Read the model definition and answer for the solid it produces. Units are mm, in the model's axes. Coordinates: 2 decimals unless noted, no trailing zeros. Order: outer loops, then holes, each group sorted by start corner. A loop starts at its lowest first (then second) coordinate and runs counter-clockwise, first axis right, second up. Notation, with made-up numbers: (31.5, -25) - (58.5, -25) arc R14 cw to (58.5, -17) - close; hole circle Ø6 at (69.5, -29). An arc over 180 degrees is marked (long way). Use one line per item in the form item = value.
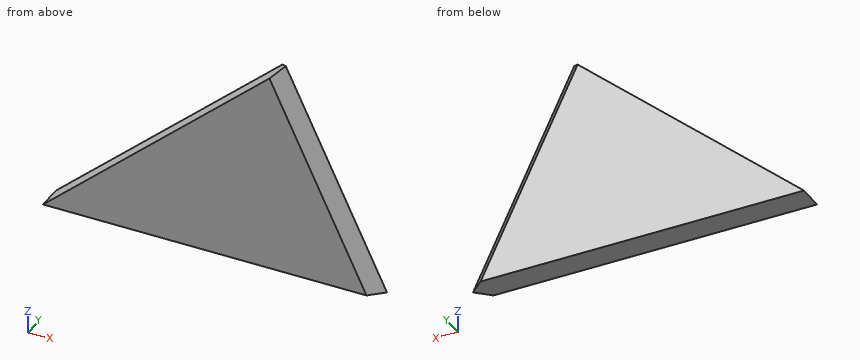
Solid Edge part; units mm, degrees
sketch "Sketch1" plane through (0, 0, 0) normal (0, -1, 0) x (1, 0, 0)
  line L0 (0, 25) -> (-28, 0)
  line L1 (-28, 0) -> (12, 0)
  line L2 (12, 0) -> (0, 25)
extrude "Protrusion1" add sketch "Sketch1" along normal mid plane 3
chamfer "Chamfer_2" distance 1.5 angle 45 2 edges at (6, 1.5, 12.5) (6, -1.5, 12.5)
(1) Straight lines are drawn through the part: L1, parallel to Z at x = -13.5, y = 0.35; L2, parallel to X at y = 0.5, z = 13.25; L3, parallel to X at y = -0.3, z = 1.75. For each, find the intervals that lie inside material, in ascending order.
Answer list:
L1 = 0 to 12.95
L2 = -13.16 to 5.09
L3 = -26.04 to 10.83
(2) Section D-D, the plane x = -14 is taken. Write down the section's boundary in (y, z), then the cut area to 3 significant figures.
Answer list:
outline = (-1.5, 0) - (1.5, 0) - (1.5, 12.5) - (-1.5, 12.5) - close
area = 37.5 mm2
(3) Section C-C, the plane y = -0.8 is taken. Write down the section's boundary in (x, z).
Answer list:
outline = (-28, 0) - (11.11, 0) - (-0.62, 24.45) - close
